Can you work these out from the model? Positions are in its coordinate system, mm. A direction names the side the tool comes from. Round coordinates to 2 decimals unless told otherwise and drop trailing zeros. Order: outer loops, then holes, each group sorted by start corner. A loop starts at its lowest first (then second) coordinate and runs counter-clockwise, first axis right, second up. Notation, with made-up numbers: M -26.75,20 L -10.75,20 A21 cw -10.75,29 Z; hole C 5,60 d6. An arc over 180 degrees is marked long. Answer as a JSON object with one key per item and string values. Group by question number.
```python
from build123d import *

# Parameters (mm, degrees)
SALIENTE_EXTRUIR1_DEPTH    = 2
SALIENTE_EXTRUIR2_DEPTH    = 4
CROQUIS2_R                 = 1.65
SALIENTE_EXTRUIR3_DEPTH    = 30
CORTAR_EXTRUIR1_DEPTH      = 27.925824036
CORTAR_EXTRUIR1_DEPTH_BACK = 27.925824036
CROQUIS3_W                 = 6.1
CROQUIS3_H                 = 6.964101615
CORTAR_EXTRUIR3_START      = -30
CROQUIS2_3_R               = 2.5
CROQUIS2_3_R_2             = 1.65
CORTAR_EXTRUIR3_DEPTH      = 5.9


with BuildPart() as part:
    # Croquis1 → Saliente-Extruir1 (new body)
    with BuildSketch(Plane.XY):
        with BuildLine():
            Line((-6, 12.05), (-11.55, 12.05))
            ThreePointArc((-11.55, 12.05), (-12.257106781, 11.757106781), (-12.55, 11.05))
            Line((-12.55, 11.05), (-12.55, -11.05))
            ThreePointArc((-12.55, -11.05), (-12.257106781, -11.757106781), (-11.55, -12.05))
            Line((-11.55, -12.05), (11.55, -12.05))
            ThreePointArc((11.55, -12.05), (12.257106781, -11.757106781), (12.55, -11.05))
            Line((12.55, -11.05), (12.55, 11.05))
            ThreePointArc((12.55, 11.05), (12.257106781, 11.757106781), (11.55, 12.05))
            Line((11.55, 12.05), (6, 12.05))
            Line((6, 12.05), (6, -8.05))
            Line((6, -8.05), (-6, -8.05))
            Line((-6, -8.05), (-6, 12.05))
        make_face()
    extrude(amount=SALIENTE_EXTRUIR1_DEPTH)

    # Croquis1<3> → Saliente-Extruir2 (add)
    with BuildSketch(Plane.XY):
        with BuildLine():
            Line((-12, 15), (12, 15))
            ThreePointArc((12, 15), (14.121320344, 14.121320344), (15, 12))
            Line((15, 12), (15, -15))
            Line((15, -15), (-15, -15))
            Line((-15, -15), (-15, 12))
            ThreePointArc((-15, 12), (-14.121320344, 14.121320344), (-12, 15))
        make_face()
        with BuildLine():
            Line((-11.55, 12.05), (11.55, 12.05))
            ThreePointArc((11.55, 12.05), (12.257106781, 11.757106781), (12.55, 11.05))
            Line((12.55, 11.05), (12.55, -11.05))
            ThreePointArc((12.55, -11.05), (12.257106781, -11.757106781), (11.55, -12.05))
            Line((11.55, -12.05), (-11.55, -12.05))
            ThreePointArc((-11.55, -12.05), (-12.257106781, -11.757106781), (-12.55, -11.05))
            Line((-12.55, -11.05), (-12.55, 11.05))
            ThreePointArc((-12.55, 11.05), (-12.257106781, 11.757106781), (-11.55, 12.05))
        make_face(mode=Mode.SUBTRACT)
    extrude(amount=SALIENTE_EXTRUIR2_DEPTH)

    # Croquis2 → Saliente-Extruir3 (add)
    with BuildSketch(Plane(origin=(15, 0, 0), x_dir=(0, 0, -1), z_dir=(1, 0, 0))):
        with BuildLine():
            Line((0, -15.035898385), (0, -15))
            Line((0, -15), (-4, -15))
            Line((-4, -15), (-4, -18.5))
            ThreePointArc((-4, -18.5), (1.791287847, -21.145751311), (0, -15.035898385))
        make_face()
        with Locations(Location((-0.5, -18.5, 0), (0, 0, 90))):
            Circle(CROQUIS2_R, mode=Mode.SUBTRACT)
    extrude(amount=-SALIENTE_EXTRUIR3_DEPTH)

    # Croquis3 → Cortar-Extruir1 (cut, two sides: drawn at the far end of the back side and taken through both)
    with BuildSketch(Plane.XY.offset(-CORTAR_EXTRUIR1_DEPTH_BACK)):
        with Locations((-6.05, -18.517949193)):
            Rectangle(CROQUIS3_W, CROQUIS3_H)
        with Locations((6.05, -18.517949193)):
            Rectangle(CROQUIS3_W, CROQUIS3_H)
    extrude(amount=CORTAR_EXTRUIR1_DEPTH + CORTAR_EXTRUIR1_DEPTH_BACK, mode=Mode.SUBTRACT)

    # Croquis2<3> → Cortar-Extruir3 (cut)
    with BuildSketch(Plane(origin=(15, 0, 0), x_dir=(0, 0, -1), z_dir=(1, 0, 0)).offset(CORTAR_EXTRUIR3_START)):
        with Locations(Location((-0.5, -18.5, 0), (0, 0, 180))):
            Circle(CROQUIS2_3_R)
        with Locations(Location((-0.5, -18.5, 0), (0, 0, 90))):
            Circle(CROQUIS2_3_R_2, mode=Mode.SUBTRACT)
    extrude(amount=CORTAR_EXTRUIR3_DEPTH, mode=Mode.SUBTRACT)


solid = part.part
```
1) For pin 1 (1.5 mm diameter, centred on y = 10.5, z = -2, fed in from -X); pin 2 (9 mm diameter, centred on x = 3, y = -0.5, fed in from -Z); pin 3 (2 mm diameter, centred on y = -19, z = 1.5, fed in from -X), each with a flat end and sliding along its axis, tell me the tip position at first contact or that it passes through.
2) I need wall thicknesses on line 1 along Z through (x, y) = (13.6, -18.5); line 2 along X through (y, z) = (-18, -2); line 3 along Z through (x, y) = (-12.1, -18.5). Which ranges of each line are inside material? Lowest first, please.
3) Which directions (+Z, -Z, +X, -X, +Y, -Y) give clear straight access to the entire face, cutting with the end or side of a thin tool? Please do faces 1 (the face through (7, 0, 0)), 2 (the face through (-12.265, 11.749, 2.986)), 3 (the face through (-9.1, -16, 2)).
4) We'd pull the mould along X, two halves only. Please class faces 4 (the face through (15, -5, 2)), 5 (the face through (12.249, 11.765, 2.986)), 6 (the face through (-12.09, -20.98, 0.17)), 7 (the face through (6, -15.036, 2)): +X half, -X half, draft (parallel to the pull), parting line (faces both ways), or undercut.
5) If we section it at C-C on y = -2.5: Write out the boundary of the cut face in (x, z).
6) If we section it at B-B on x = 2.5: Write out the boundary of the cut face in (y, z).
7) If we section it at A-A on z = 0.5: Count the separate pieces of the cut face and the enclosed holes in it, plus the area to 3 significant figures.
8) If we section it at D-D on x = -10.75: Write out the boundary of the cut face in (y, z).
Findings:
{
 "1": {"pin 1": "passes through", "pin 2": "stops at z = 0", "pin 3": "stops at x = -3"},
 "2": {"line 1": "z = -3 to -1.15, 2.15 to 4", "line 2": "x = -15 to -9.1, -3 to 3, 9.1 to 15", "line 3": "z = -3 to -2, 3 to 4"},
 "3": {"face 1": "-Z, +X, -X, +Y", "face 2": "+Z", "face 3": "+Z, -Z, -Y"},
 "4": {"face 4": "+X half", "face 5": "undercut", "face 6": "draft", "face 7": "undercut"},
 "5": {"outline": "M -15,0 L -6,0 L -6,2 L -12.55,2 L -12.55,4 L -15,4 Z; M 6,0 L 15,0 L 15,4 L 12.55,4 L 12.55,2 L 6,2 Z"},
 "6": {"outline": "M -18.5,4 A3.5 ccw long -15.04,0 L -8.05,0 L -8.05,2 L -12.05,2 L -12.05,4 Z; M 12.05,0 L 15,0 L 15,4 L 12.05,4 Z; hole C -18.5,0.5 d3.3"},
 "7": {"separate pieces": "4", "enclosed holes": "1", "area": "711 mm^2"},
 "8": {"outline": "M -18.5,4 A3.5 ccw long -15.04,0 L 15,0 L 15,4 L 12.05,4 L 12.05,2 L -12.05,2 L -12.05,4 Z; hole C -18.5,0.5 d5"}
}
